The listing builds one solid part. Answer for the finished solid, in the listing's coordinates (mm). A direction names the side the tool comes from. Coordinates: 2 decimals unless noted, no trailing zeros. Write each loop counter-clockwise with the first axis right and the second up, starting at its lowest first coordinate (ties: lowest second). Pieces come first, ordered by that corner, then holes.
(1) The part is cut by section A-A on x = 0. Determine the outline of the cut face in (y, z).
(2) Straight lines are drawn through the part: line 1 (Z direction, x = 0, y = -2.35); line 2 (X direction, y = 22.5, z = 5); line 3 (X direction, y = 5.5, z = 7.25). For each, find the intervals that lie inside material, in ascending order.
(3) The part is cut by section D-D on x = -5.5. Determine the outline of the cut face in (y, z), plus the area to 3 significant figures.
(4) Given P1, Ø6, axis at x = 0, z = 5, coming from the -Y side; P2, Ø3, axis at x = 2, z = 6.5, coming from the +Y side; P3, Ø4, axis at y = 28.83, z = 5, coming from the +X side; P4, Ø1, axis at x = 0.5, z = 6.5, coming from the +Y side, each flat-ended and moving along its own axis, determine where each tip first touches the part or whether it passes through.
(5) For a pull along Z with two mould halves and no side action, classify faces 1 (the flat face through (0, -6, 1.5)), 2 (the flat face through (-17, 3, 5)), 3 (the flat face through (0, -5, 0)) as +Z half, -Z half, draft (parallel to the pull), parting line (faces both ways), or undercut.
(6) The part is cut by section B-B on y = 2. Determine the outline of the cut face in (x, z).
(7) Which of the six approach directions +Z, -Z, +X, -X, +Y, -Y give full straight-line access (tool end or side, diameter ignored) to faces 4 (the flat face through (20, 23, 8.5)), 5 (the flat face through (19, 21.3, 0.5)), 6 (the flat face through (-22, 29, 5))?
(8) The part is cut by section C-C on z = 5. Give the number of separate pieces and of enclosed holes in the cut face, plus the area to 3 significant figures.
from build123d import *

# Parameters (mm, degrees)
BOSS_EXTRUDE1_DEPTH            = 10
SKETCH2_R                      = 2.5
CUT_EXTRUDE1_DEPTH             = 3
CUT_EXTRUDE1_DIRECTION_2_REACH = 62.498
CUT_EXTRUDE2_DEPTH             = 3
CUT_EXTRUDE3_REACH             = 56.268
SKETCH4_R                      = 2.5
SKETCH5_W                      = 38
SKETCH5_H                      = 7
CUT_EXTRUDE4_DEPTH             = 4


with BuildPart() as part:
    # Sketch1 → Boss-Extrude1 (new body)
    with BuildSketch(Plane.XY):
        Polygon((-27, 38), (-19, 38), (-19, 5), (-14, 0), (14, 0), (19, 5), (19, 38), (27, 38), (27, -3), (22, -8), (-22, -8), (-27, -3), align=None)
    extrude(amount=BOSS_EXTRUDE1_DEPTH)

    # Sketch2 → Cut-Extrude1 (cut)
    with BuildSketch(Plane(origin=(-19, 0, 0), x_dir=(0, 0, -1), z_dir=(1, 0, 0))):
        with Locations(Location((-5, 28.83, 0), (0, 0, 90))):
            Circle(SKETCH2_R)
    extrude(amount=-CUT_EXTRUDE1_DEPTH, mode=Mode.SUBTRACT)

    # Sketch2 → Cut-Extrude1 direction 2 (cut, up to next)
    with BuildSketch(Plane(origin=(-19, 0, 0), x_dir=(0, 0, -1), z_dir=(1, 0, 0)), mode=Mode.PRIVATE) as cut_extrude1_direction_2_sk1:
        with Locations(Location((-5, 28.83, 0), (0, 0, 90))):
            Circle(SKETCH2_R)
    cut_extrude1_direction_2_tool1 = extrude(cut_extrude1_direction_2_sk1.sketch, amount=CUT_EXTRUDE1_DIRECTION_2_REACH, mode=Mode.PRIVATE) & part.part
    add(cut_extrude1_direction_2_tool1.solids().sort_by_distance((-19, 28.83, 5))[0], mode=Mode.SUBTRACT)

    # Sketch3 → Cut-Extrude2 (cut)
    with BuildSketch(Plane.ZY.offset(-19)):
        with BuildLine():
            Line((8.5, 28.503575447), (8.5, 16.503575447))
            ThreePointArc((8.5, 16.503575447), (5, 13.003575447), (1.5, 16.503575447))
            Line((1.5, 16.503575447), (1.5, 28.503575447))
            ThreePointArc((1.5, 28.503575447), (5, 32.003575447), (8.5, 28.503575447))
        make_face()
    extrude(amount=-CUT_EXTRUDE2_DEPTH, mode=Mode.SUBTRACT)

    # Sketch4 → Cut-Extrude3 (cut, up to next)
    with BuildSketch(Plane.XZ.offset(8), mode=Mode.PRIVATE) as cut_extrude3_sk1:
        with Locations((0, 5)):
            Circle(SKETCH4_R)
    cut_extrude3_tool1 = extrude(cut_extrude3_sk1.sketch, amount=-CUT_EXTRUDE3_REACH, mode=Mode.PRIVATE) & part.part
    add(cut_extrude3_tool1.solids().sort_by_distance((0, -8, 5))[0], mode=Mode.SUBTRACT)

    # Sketch5 → Cut-Extrude4 (cut)
    with BuildSketch(Plane.XZ.offset(8)):
        with Locations((0, 5)):
            Rectangle(SKETCH5_W, SKETCH5_H)
    extrude(amount=-CUT_EXTRUDE4_DEPTH, mode=Mode.SUBTRACT)


solid = part.part
Model answer:
1. outline: (-8, 0) - (0, 0) - (0, 2.5) - (-4, 2.5) - (-4, 1.5) - (-8, 1.5) - close; (-8, 8.5) - (-4, 8.5) - (-4, 7.5) - (0, 7.5) - (0, 10) - (-8, 10) - close
2. line 1: z = 0 to 2.5, 7.5 to 10
2. line 2: x = -27 to -19, 22 to 27
2. line 3: x = -27 to -19, 19 to 27
3. outline: (-8, 0) - (0, 0) - (0, 10) - (-8, 10) - (-8, 8.5) - (-4, 8.5) - (-4, 1.5) - (-8, 1.5) - close
3. area: 52.0 mm2
4. P1: stops at y = -4
4. P2: stops at y = 0
4. P3: stops at x = -22
4. P4: passes through
5. face 1: undercut
5. face 2: draft
5. face 3: -Z half
6. outline: (-27, 0) - (-16, 0) - (-16, 10) - (-27, 10) - close; (16, 0) - (27, 0) - (27, 10) - (16, 10) - close
7. face 4: none
7. face 5: +Z, -Z, +Y
7. face 6: +X
8. separate pieces: 3
8. enclosed holes: 0
8. area: 771 mm2
